Design review of the part built by this model. Coordinates are the model's own, in mm. Face numbers are marked on the shaded views. Give positions to 0.01 mm unless a question says otherwise; leave off trailing zeros. Order: outer loops, then holes, each group sorted by start corner. A loop starts at its lowest first (then second) coordinate and runs counter-clockwise, first axis right, second up. Notation, with made-up numbers: (11, -20) -> (67, -20) arc R13 cw to (67, 1) -> close; hole circle Ø2 at (-15.75, 80). An arc over 180 degrees is marked (long way). Use a Markdown table: item, result. Add a question column.
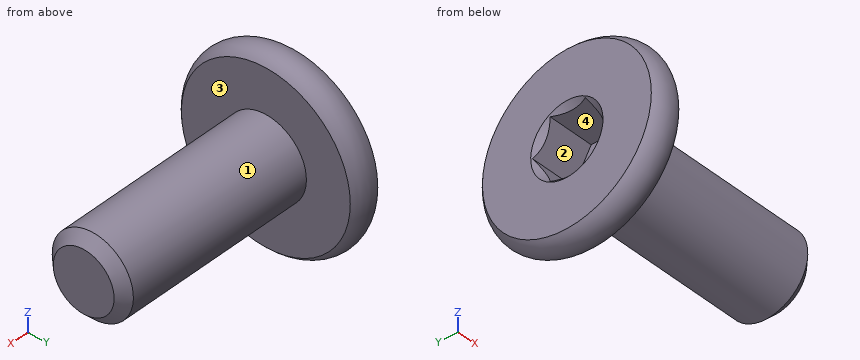
```python
from build123d import *

# Parameters (mm, degrees)
SKETCH2_R           = 2
BOSS_EXTRUDE1_DEPTH = 10
CHAMFER1_SIZE       = 0.5
CUT_EXTRUDE1_DEPTH  = 2.3
SKETCH8_R           = 1.782050808
CUT_EXTRUDE2_DEPTH  = 1
CUT_EXTRUDE2_TAPER  = 45


with BuildPart() as part:
    # Sketch2 → Boss-Extrude1 (new body)
    with BuildSketch(Plane(origin=(0, 0, 0), x_dir=(0, 0, -1), z_dir=(1, 0, 0))):
        Circle(SKETCH2_R)
    extrude(amount=-BOSS_EXTRUDE1_DEPTH)

    # Chamfer1
    chamfer1_edges = [part.edges().sort_by_distance(p)[0] for p in [
        (0, 0, 2),
    ]]
    chamfer(chamfer1_edges, length=CHAMFER1_SIZE)

    # Sketch6 → Revolve1 (revolve)
    with BuildSketch(Plane.XY):
        with BuildLine():
            Line((-11.5, 0), (-11.5, 4.161437828))
            ThreePointArc((-11.5, 4.161437828), (-10.75, 4.5), (-10, 4.161437828))
            Line((-10, 4.161437828), (-10, 0))
            Line((-10, 0), (-11.5, 0))
        make_face()
    revolve(axis=Axis((-10, 0, 0), (-1, 0, 0)))

    # Sketch7 → Cut-Extrude1 (cut)
    with BuildSketch(Plane.ZY.offset(11.5)):
        Polygon((0, 1.732050808), (-1.5, 0.866025404), (-1.5, -0.866025404), (0, -1.732050808), (1.5, -0.866025404), (1.5, 0.866025404), align=None)
    extrude(amount=-CUT_EXTRUDE1_DEPTH, mode=Mode.SUBTRACT)

    # Sketch8 → Cut-Extrude2 (cut)
    with BuildSketch(Plane.ZY.offset(11.5)):
        Circle(SKETCH8_R)
    extrude(amount=-CUT_EXTRUDE2_DEPTH, taper=CUT_EXTRUDE2_TAPER, mode=Mode.SUBTRACT)


solid = part.part
```
1) Add section B-B (x = -3.25). Give the boundary of the cut face in (y, z), then the cut area to 3 significant figures.
2) Add section A-A (x = -10.25). Give the boundary of the cut face in (y, z), then the cut area to 3 significant figures.
3) The part is to be moulded in two halves that separate along Y. For the marked faces 1, 2, 3 and 4, say which applies: +Y half, -Y half, draft (parallel to the pull), parting line (faces both ways), or undercut.
4) For L1, parallel to X at y = 2.5, z = 0; L2, parallel to X at y = -0.75, z = 0.5; L3, parallel to Y at x = -3.5, z = -1, list the stretches that pass through material, from the lowest coordinate up. Write a range as [from, to].
5) Insertion check: pin 1 (2 mm diameter, centred on x = -10, y = 1, fed in from -Z); pin 2 (3 mm diameter, centred on x = -5, z = -1.5, fed in from -Y); pin 3 (0.9 mm diameter, centred on y = -0.5, z = -0.5, fed in from -X). Each pin has a flat end and moves straight along its axis. Give the tip position at first contact, or say it passes through.
Worked answers:
| question | item | result |
|---|---|---|
| 1 | outline | circle Ø4 at (0, 0) |
| 1 | area | 12.6 mm^2 |
| 2 | outline | circle Ø8.73 at (0, 0); hole (-1.73, 0) -> (-0.87, -1.5) -> (0.87, -1.5) -> (1.73, 0) -> (0.87, 1.5) -> (-0.87, 1.5) -> close |
| 2 | area | 52.1 mm^2 |
| 3 | face 1 | parting line |
| 3 | face 2 | undercut |
| 3 | face 3 | draft |
| 3 | face 4 | undercut |
| 4 | L1 | [-11.5, -10] |
| 4 | L2 | [-9.2, 0] |
| 4 | L3 | [-1.73, 1.73] |
| 5 | pin 1 | z = -4.49 |
| 5 | pin 2 | y = -2 |
| 5 | pin 3 | x = -9.2 |
